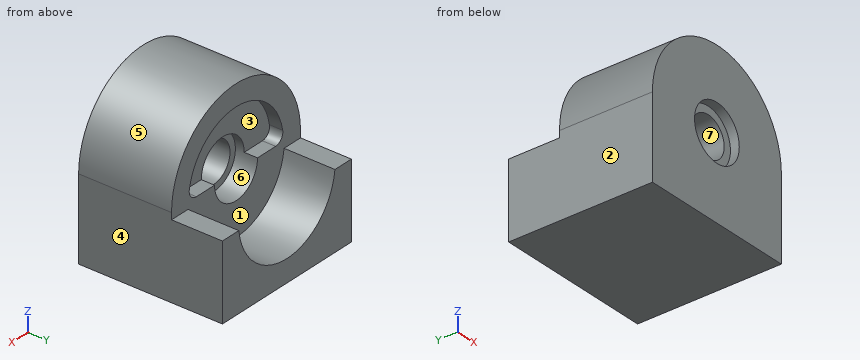
from build123d import *

# Parameters (mm, degrees)
F1_DEPTH  = 65
F2_R      = 12.5
F2_R_2    = 9
F3_DEPTH  = 4
F4_W      = 23
F4_H      = 40
F4_H_2    = 3
F5_DEPTH  = 72
F7_DEPTH  = 23
F8_R      = 12
F8_R_2    = 9
F9_DEPTH  = 10
F11_DEPTH = 6


with BuildPart() as f1:
    # F0 (on Front) → F1 (new body)
    with BuildSketch(Plane.XZ):
        with BuildLine():
            Line((36, 0), (9, 0))
            ThreePointArc((9, 0), (0, -9), (-9, 0))
            Line((-9, 0), (-36, 0))
            ThreePointArc((-36, 0), (0, -36), (36, 0))
        make_face()
        with BuildLine():
            ThreePointArc((-9, 0), (0, 9), (9, 0))
            Line((9, 0), (36, 0))
            ThreePointArc((36, 0), (0, 36), (-36, 0))
            Line((-36, 0), (-9, 0))
        make_face()
        with BuildLine():
            Line((36, -37), (36, 0))
            ThreePointArc((36, 0), (0, -36), (-36, 0))
            Line((-36, 0), (-36, -37))
            Line((-36, -37), (36, -37))
        make_face()
    extrude(amount=F1_DEPTH)

    # F2 (on face) → F3 (cut)
    with BuildSketch(Plane.XZ.offset(65)):
        Circle(F2_R)
        Circle(F2_R_2, mode=Mode.SUBTRACT)
    extrude(amount=-F3_DEPTH, mode=Mode.SUBTRACT)

    # F4 (on face) → F5 (cut)
    with BuildSketch(Plane.YZ.offset(36)):
        with Locations((-11.5, 20)):
            Rectangle(F4_W, F4_H)
        with Locations((-11.5, -1.5)):
            Rectangle(F4_W, F4_H_2)
    extrude(amount=-F5_DEPTH, mode=Mode.SUBTRACT)

    # F6 (on face) → F7 (cut)
    with BuildSketch(Plane(origin=(0, 0, 0), x_dir=(-1, 0, 0), z_dir=(0, 1, 0))):
        with BuildLine():
            ThreePointArc((26.83281573, -3), (26.9581715321, -1.5023274094), (27, 0))
            ThreePointArc((27, 0), (-1.5023274094, 26.9581715321), (-26.83281573, -3))
            Line((-26.83281573, -3), (-8.4852813742, -3))
            ThreePointArc((-8.4852813742, -3), (0, -9), (8.4852813742, -3))
            Line((8.4852813742, -3), (26.83281573, -3))
        make_face()
        with BuildLine():
            Line((-8.4852813742, -3), (-26.83281573, -3))
            ThreePointArc((-26.83281573, -3), (0, -27), (26.83281573, -3))
            Line((26.83281573, -3), (8.4852813742, -3))
            ThreePointArc((8.4852813742, -3), (0, -9), (-8.4852813742, -3))
        make_face()
    extrude(amount=-F7_DEPTH, mode=Mode.SUBTRACT)

    # F8 (on face) → F9 (cut)
    with BuildSketch(Plane(origin=(0, -23, 0), x_dir=(-1, 0, 0), z_dir=(0, 1, 0))):
        Circle(F8_R)
        Circle(F8_R_2, mode=Mode.SUBTRACT)
    extrude(amount=-F9_DEPTH, mode=Mode.SUBTRACT)

    # F10 (on face) → F11 (cut)
    with BuildSketch(Plane(origin=(0, -23, 0), x_dir=(-1, 0, 0), z_dir=(0, 1, 0))):
        with BuildLine():
            ThreePointArc((22.1415898255, 0), (25.2111536743, 1.4352821251), (26.0778724611, 4.7111111111))
            ThreePointArc((26.0778724611, 4.7111111111), (0, 26.5), (-26.0778724611, 4.7111111111))
            ThreePointArc((-26.0778724611, 4.7111111111), (-25.2111536743, 1.4352821251), (-22.1415898255, 0))
            Line((-22.1415898255, 0), (-12, 0))
            ThreePointArc((-12, 0), (0, 12), (12, 0))
            Line((12, 0), (22.1415898255, 0))
        make_face()
    extrude(amount=-F11_DEPTH, mode=Mode.SUBTRACT)


solid = f1.part
Part model, mm, in its own coordinate system. Face numbers are marked on the shaded views. A direction names the side the tool comes from. Coordinates: 2 decimals unless noted, no trailing zeros. Order: outer loops, then holes, each group sorted by start corner. A loop starts at its lowest first (then second) coordinate and runs counter-clockwise, first axis right, second up. Notation, with made-up numbers: M -16.75,20 L 16.25,20 A27 cw 16.25,49 Z; hole C -36.5,20 d7. An arc over 180 degrees is marked long. One line per question, with ' | ' between items.
Q1. Two-plate mould, pull along Z, no slides. Class the marked faces 4, 5, 6 and 7: +Z half, -Z half, draft (parallel to the pull), parting line (faces both ways), or undercut.
A:
face 4: draft | face 5: +Z half | face 6: undercut | face 7: undercut
Q2. Slice it at D-D (y = -4.5). Give the cut face in (x, z).
A:
outline: M -36,-37 L 36,-37 L 36,-3 L 26.83,-3 A27 cw -26.83,-3 L -36,-3 Z
Q3. Slice it at B-B (y = -27). Give the cut face in (x, z), and give its area (3 significant figures).
A:
outline: M -36,-37 L 36,-37 L 36,0 A36 ccw -36,0 Z; hole M -26.08,4.71 A4 ccw -22.14,0 L -12,0 A12 ccw 12,0 L 22.14,0 A4 ccw 26.08,4.71 A26.5 ccw Z | area: 3,380 mm^2
Q4. Slice it at C-C (z = -5). Give the cut face in (x, y).
A:
outline: M -36,-65 L -11.46,-65 L -11.46,-61 L -7.48,-61 L -7.48,-33 L -10.91,-33 L -10.91,-23 L -26.53,-23 L -26.53,0 L -36,0 Z; M 7.48,-61 L 11.46,-61 L 11.46,-65 L 36,-65 L 36,0 L 26.53,0 L 26.53,-23 L 10.91,-23 L 10.91,-33 L 7.48,-33 Z
Q5. Drill centre lines: line 1 (Z direction, x = 0, y = -30.25); line 2 (Z direction, x = 0, y = -40.25); line 3 (Y direction, x = -11.5, z = -15). Where is each one in solid material? Low to high.
A:
line 1: z = -37 to -12, 12 to 36 | line 2: z = -37 to -9, 9 to 36 | line 3: y = -65 to -23
Q6. Pin check, flat tips, straight feed: P1, Ø5, axis at x = 17, y = -26, coming from the +Z side; P2, Ø20.5, axis at x = 0, z = 0, coming from the +Y side; P3, Ø1, axis at x = 26.5, y = -44.5, coming from the +Z side. Stop position of each tip, or through.
A:
P1: stops at z = 32.95 | P2: stops at y = -33 | P3: stops at z = 24.9
Q7. 3-axis set-ups, long thin cutter, end or side, ignore diameter. For the marked faces 1, 2 and 3: which of +Z, -Z, +X, -X, +Y, -Y reach the whole face in a straight line?
A:
face 1: +Z, +Y | face 2: +Z, -Z, -X, +Y, -Y | face 3: +Y
Q8. Slice it at A-A (x = 0). Give the cut face in (y, z).
A:
outline: M -65,-37 L 0,-37 L 0,-27 L -23,-27 L -23,-12 L -33,-12 L -33,-9 L -61,-9 L -61,-12.5 L -65,-12.5 Z; M -65,12.5 L -61,12.5 L -61,9 L -33,9 L -33,12 L -29,12 L -29,26.5 L -23,26.5 L -23,36 L -65,36 Z
